```python
from build123d import *

# Parameters (mm, degrees)
F0_R     = 39.32561
F1_DEPTH = 25.4
F3_DEPTH = 25.4
F5_DEPTH = 25.4
F7_DEPTH = 25.4


with BuildPart() as f1:
    # F0 (on Front) → F1 (new body)
    with BuildSketch(Plane.XZ):
        with Locations((0, 58.036841)):
            Circle(F0_R)
    extrude(amount=F1_DEPTH)

    # F2 (on Front) → F3 (join)
    with BuildSketch(Plane.XZ):
        Polygon((20.801723, 23.11036), (-15.714049, 23.506835), (-15.714049, -76.474115), (20.801723, -76.474115), align=None)
    extrude(amount=F3_DEPTH)

    # F4 (on Front) → F5 (join)
    with BuildSketch(Plane.XZ):
        Polygon((-11.353261, 0), (-15.755951, 11.085525), (-53.817809, -29.885441), (-45.926862, -37.216098), align=None)
        Polygon((52.584887, -25.371686), (20.5549, 8.637682), (16.058708, 0), (45.89106, -31.675924), align=None)
    extrude(amount=F5_DEPTH)

    # F6 (on Front) → F7 (join)
    with BuildSketch(Plane.XZ):
        Polygon((-12.695789, -69.341376), (-14.400601, -78.842267), (-38.887709, -115.700036), (-15.157491, -115.700036), (0, -81.533164), (0, -69.341376), align=None)
        Polygon((6.92448, -69.341376), (0, -69.341376), (0, -81.533164), (18.049568, -115.125895), (40.677667, -115.125895), (17.291129, -69.341376), align=None)
    extrude(amount=F7_DEPTH)


solid = f1.part
```
Geometry check sheet. Reference: the model listing, model coordinates, mm. A direction names the side the tool comes from. Round coordinates to 2 decimals unless told otherwise and drop trailing zeros. Order: outer loops, then holes, each group sorted by start corner. A loop starts at its lowest first (then second) coordinate and runs counter-clockwise, first axis right, second up. Notation, with made-up numbers: (-31, 13.25) - (25, 13.25) arc R32 ccw to (25, 40.25) - close; hole circle Ø2 at (-15, 10.5). An arc over 180 degrees is marked (long way). Use a Markdown table: item, result. Add a question column.
(1) Tool access check on faces 5 (the flat face through (-7.685, -12.522, -98.856)), 6 (the flat face through (-26.47, -12.52, -97.01)), 7 (the flat face through (36.916, -12.522, -8.734)), 8 (the flat face through (-31.03, -12.52, -21.18)), 9 (the flat face through (29, -13, -115.126)). Record the directions out of +Z, -Z, +X, -X, +Y, -Y that give a thin tool (end or side, any length) a straight path to the whole face; none if there is none.
(2) Sectioned sample at B-B, the plane z = -95.5. Enter the section's corners in (x, y).
(3) Sectioned sample at D-D, the plane z = -42. Enter the section's corners in (x, y), and give its area (4 significant figures).
(4) Sectioned sample at A-A, the plane y = -14.25. Enter the section's corners in (x, z), and give its area (3 significant figures).
(5) Depth check by flat-ended pin: pin 1 (1 mm diameter, centred on x = 4, y = -17, fed in from -Z); pin 2 (12 mm diameter, centred on x = 13, y = -12, fed in from +Z); pin 3 (6 mm diameter, centred on y = -12, z = -56.5, fed in from +X); pin 4 (1 mm diameter, centred on x = -17, z = -79, fed in from -Y). Enter the tip coordinate at first touch or a pass-through.
(6) Release check for a two-part mould opening along Z. For faces 1 (the flat face through (-1, 0, -8)), 2 (the flat face through (49.19, -12.52, -28.57)), 3 (the flat face through (-15.714, -13, -40)), 4 (the flat face through (20.802, -13, -41)) record: pulls with the +Z half, pulls with the -Z half, needs draft (parallel to the pull), parting line crosses it, or undercut.
(7) Sectioned sample at C-C, the plane x = -32. Enter the section's corners in (y, z), and give its area (3 significant figures).
(8) Material ranges on line 1 along X through (y, z) = (-13.5, -6); line 2 along X through (y, z) = (-9, -19.5); line 3 along Z through (x, y) = (-18, -19.25), recorded low to high. Write a range as [from, to].
Answers below:
| question | item | result |
|---|---|---|
| 1 | face 5 | -Z, +Y, -Y |
| 1 | face 6 | -X, +Y, -Y |
| 1 | face 7 | +X, +Y, -Y |
| 1 | face 8 | +Y, -Y |
| 1 | face 9 | -Z, +X, +Y, -Y |
| 2 | outline | (-25.47, -25.4) - (-6.2, -25.4) - (-6.2, 0) - (-25.47, 0) - close; (7.5, -25.4) - (30.65, -25.4) - (30.65, 0) - (7.5, 0) - close |
| 3 | outline | (-15.71, -25.4) - (20.8, -25.4) - (20.8, 0) - (-15.71, 0) - close |
| 3 | area | 927.5 mm² |
| 4 | outline | (-53.82, -29.89) - (-45.93, -37.22) - (-15.71, -4.69) - (-15.71, -76.47) - (-13.98, -76.47) - (-14.4, -78.84) - (-38.89, -115.7) - (-15.16, -115.7) - (0, -81.53) - (18.05, -115.13) - (40.68, -115.13) - (20.8, -76.21) - (20.8, -5.04) - (45.89, -31.68) - (52.58, -25.37) - (20.8, 8.38) - (20.8, 23.11) - (18.13, 23.14) arc R39.33 ccw (long way) to (-15.71, 21.99) - (-15.71, 10.98) - (-15.76, 11.09) - close |
| 4 | area | 11,000 mm² |
| 5 | pin 1 | z = -89.91 |
| 5 | pin 2 | z = 96.73 |
| 5 | pin 3 | x = 20.8 |
| 5 | pin 4 | through |
| 6 | face 1 | needs draft |
| 6 | face 2 | pulls with the -Z half |
| 6 | face 3 | undercut |
| 6 | face 4 | undercut |
| 7 | outline | (-25.4, -115.7) - (0, -115.7) - (0, -105.33) - (-25.4, -105.33) - close; (-25.4, -22.22) - (0, -22.22) - (0, -6.4) - (-25.4, -6.4) - close; (-25.4, 35.18) - (0, 35.18) - (0, 80.9) - (-25.4, 80.9) - close |
| 7 | area | 1,830 mm² |
| 8 | line 1 | [-31.63, -16.93], [-15.71, 20.8], [21.71, 34.34] |
| 8 | line 2 | [-44.17, -29.47], [-15.71, 20.8], [34.42, 47.05] |
| 8 | line 3 | [-115.7, -84.26], [-7.15, 8.67], [23.07, 93] |
